```python
from build123d import *

# Parameters (mm, degrees)
SKETCH1_R           = 2.8
BOSS_EXTRUDE1_DEPTH = 1.5
SKETCH2_R           = 2.25
BOSS_EXTRUDE2_DEPTH = 7
SKETCH3_R           = 2.25
BOSS_EXTRUDE3_DEPTH = 15
CUT_EXTRUDE1_DEPTH  = 13.8
CUT_EXTRUDE2_DEPTH  = 13.8
SKETCH6_R           = 1.75
CUT_EXTRUDE3_DEPTH  = 26.0000001


with BuildPart() as part:
    # Sketch1 → Boss-Extrude1 (new body)
    with BuildSketch(Plane(origin=(0, 0, 0), x_dir=(1, 0, 0), z_dir=(0, 1, 0))):
        Circle(SKETCH1_R)
    extrude(amount=BOSS_EXTRUDE1_DEPTH)

    # Sketch2 → Boss-Extrude2 (add)
    with BuildSketch(Plane(origin=(0, 1.5, 0), x_dir=(1, 0, 0), z_dir=(0, 1, 0))):
        Circle(SKETCH2_R)
    extrude(amount=BOSS_EXTRUDE2_DEPTH)

    # Sketch3 → Boss-Extrude3 (add)
    with BuildSketch(Plane.XZ):
        Circle(SKETCH3_R)
    extrude(amount=BOSS_EXTRUDE3_DEPTH)

    # Sketch4 → Cut-Extrude1 (cut, through all)
    with BuildSketch(Plane.XY.offset(10)):
        with BuildLine():
            Line((-0.5, 6), (-0.5, 8.5))
            ThreePointArc((-0.5, 8.5), (0, 9), (0.5, 8.5))
            Line((0.5, 8.5), (0.5, 6))
            ThreePointArc((0.5, 6), (0, 5.5), (-0.5, 6))
        make_face()
        with BuildLine():
            Line((0.5, -11.5), (0.5, -15))
            ThreePointArc((0.5, -15), (0, -15.5), (-0.5, -15))
            Line((-0.5, -15), (-0.5, -11.5))
            ThreePointArc((-0.5, -11.5), (0, -11), (0.5, -11.5))
        make_face()
    extrude(amount=-CUT_EXTRUDE1_DEPTH, mode=Mode.SUBTRACT)

    # Sketch5 → Cut-Extrude2 (cut, through all)
    with BuildSketch(Plane(origin=(10, 0, 0), x_dir=(0, 0, -1), z_dir=(1, 0, 0))):
        with BuildLine():
            Line((0.5, -4), (0.5, -10))
            ThreePointArc((0.5, -10), (0, -10.5), (-0.5, -10))
            Line((-0.5, -10), (-0.5, -4))
            ThreePointArc((-0.5, -4), (0, -3.5), (0.5, -4))
        make_face()
    extrude(amount=-CUT_EXTRUDE2_DEPTH, mode=Mode.SUBTRACT)

    # Sketch6 → Cut-Extrude3 (cut, through all)
    with BuildSketch(Plane(origin=(0, 10, 0), x_dir=(1, 0, 0), z_dir=(0, 1, 0))):
        Circle(SKETCH6_R)
    extrude(amount=-CUT_EXTRUDE3_DEPTH, mode=Mode.SUBTRACT)


solid = part.part
```
Input: part model. Units: mm. Frame: model coordinates. A direction names the side the tool comes from. Coordinates: 2 decimals unless noted, no trailing zeros. Loops run counter-clockwise (first coordinate to the right, second up) from the corner with the lowest first, then second, coordinate; pieces in that order, holes last. Notation, with made-up numbers: (37.25, 16.5) -> (84.25, 16.5) arc R19 ccw to (84.25, 25.5) -> close; hole circle Ø1 at (87, 33). An arc over 180 degrees is marked (long way). Use a Markdown table: item, result.
1) Pull-direction query (X, two-part tool) for faces 3 (the cylindrical face through (2.146, -7.395, 0.676)), 4 (the cylindrical face through (1.669, -3.085, -0.526)), 5 (the flat face through (2, -15, 0)); classes: released by +X, released by -X, zero draft, split by the parting line, or undercut.
Results found:
| item | result |
|---|---|
| face 3 | split by the parting line |
| face 4 | undercut |
| face 5 | zero draft |
2) Cut plane A-A (x = 0). Return the cut outline in (y, z).
Results found:
| item | result |
|---|---|
| outline | (-11, -2.25) -> (0, -2.25) -> (0, -2.8) -> (1.5, -2.8) -> (1.5, -2.25) -> (5.5, -2.25) -> (5.5, -1.75) -> (-11, -1.75) -> close; (-11, 1.75) -> (5.5, 1.75) -> (5.5, 2.25) -> (1.5, 2.25) -> (1.5, 2.8) -> (0, 2.8) -> (0, 2.25) -> (-11, 2.25) -> close |
3) Cut plane C-C (y = -8.75). Return the cut outline in (x, z), then the cut area to 3 significant figures.
Results found:
| item | result |
|---|---|
| outline | (-2.19, -0.5) arc R2.25 ccw to (2.19, -0.5) -> (1.68, -0.5) arc R1.75 cw to (-1.68, -0.5) -> close; (-2.19, 0.5) -> (-1.68, 0.5) arc R1.75 cw to (1.68, 0.5) -> (2.19, 0.5) arc R2.25 ccw to start |
| area | 5.27 mm2 |
4) Contact query for flat-ended pins moving along their axis: pin 1 (0.6 mm diameter, centred on y = 7.5, z = 2, fed in from -X); pin 2 (0.6 mm diameter, centred on y = -13.5, z = -2, fed in from +X); pin 3 (3 mm diameter, centred on y = -4, z = 2, fed in from +X). Output: stop coordinate, or through.
Results found:
| item | result |
|---|---|
| pin 1 | stops at x = -1.47 |
| pin 2 | stops at x = 1.47 |
| pin 3 | stops at x = 2.19 |
5) Cut plane B-B (z = 0). Return the cut outline in (x, y), then the cut area to 4 significant figures.
Results found:
| item | result |
|---|---|
| outline | (-2.8, 0) -> (-2.25, 0) -> (-2.25, -3.5) -> (-1.75, -3.5) -> (-1.75, 8.5) -> (-2.25, 8.5) -> (-2.25, 1.5) -> (-2.8, 1.5) -> close; (-2.25, -15) -> (-1.75, -15) -> (-1.75, -10.5) -> (-2.25, -10.5) -> close; (1.75, -15) -> (2.25, -15) -> (2.25, -10.5) -> (1.75, -10.5) -> close; (1.75, -3.5) -> (2.25, -3.5) -> (2.25, 0) -> (2.8, 0) -> (2.8, 1.5) -> (2.25, 1.5) -> (2.25, 8.5) -> (1.75, 8.5) -> close |
| area | 18.15 mm2 |
6) Access query for faces 1 (the flat face through (-2, 8.5, 0)), 2 (the cylindrical face through (2.08, 4.95, 0.86)). Directions: +Z, -Z, +X, -X, +Y, -Y. A direction counts if a zero-diameter tool reaches every point of the face in a straight line with its end or side. Return the directions, or none.
Results found:
| item | result |
|---|---|
| face 1 | +Z, -Z, +X, -X, +Y |
| face 2 | +Y |
7) Cut plane D-D (z = -1.1). Return the cut outline in (x, y).
Results found:
| item | result |
|---|---|
| outline | (-2.57, 0) -> (-1.96, 0) -> (-1.96, -15) -> (-1.36, -15) -> (-1.36, 8.5) -> (-1.96, 8.5) -> (-1.96, 1.5) -> (-2.57, 1.5) -> close; (1.36, -15) -> (1.96, -15) -> (1.96, 0) -> (2.57, 0) -> (2.57, 1.5) -> (1.96, 1.5) -> (1.96, 8.5) -> (1.36, 8.5) -> close |
8) Material intervals for line 1 along Z through (x, y) = (0, -6.5); line 2 along Y through (x, z) = (1, 2.55), sorted ascending. Write a range as from..to.
Results found:
| item | result |
|---|---|
| line 1 | z = -2.25..-1.75, 1.75..2.25 |
| line 2 | y = 0..1.5 |
